Autodesk Fusion 360 part; units mm, degrees
sketch "Sketch1" plane through (0, 0, 0) normal (0, 1, 0) x (1, 0, 0)
  line L0 (4.0197, -0.419) -> (2.3727, 3.2717)
  line L1 (2.3727, 3.2717) -> (-1.647, 3.6906)
  line L2 (-1.647, 3.6906) -> (-4.0197, 0.419)
  line L3 (-4.0197, 0.419) -> (-2.3727, -3.2717)
  line L4 (-2.3727, -3.2717) -> (1.647, -3.6906)
  line L5 (1.647, -3.6906) -> (4.0197, -0.419)
  circle A0 centre (0, 0) radius 3.5
  dimension "d2" = 7
extrude "Extrude1" add sketch "Sketch1" along normal blind 2.5
sketch "Sketch2" plane through (0, 0, 0) normal (0, 1, 0) x (1, 0, 0)
  circle A0 centre (0, 0) radius 5
  dimension "d5" = 10
extrude "Extrude2" add sketch "Sketch2" against normal blind 0.5
sketch "Sketch3" plane through (0, 2.5, 0) normal (0, 1, 0) x (-1, 0, 0)
  line L0 (-1.647, 3.6906) -> (-4.0197, 0.419)
  line L1 (-4.0197, 0.419) -> (-2.3727, -3.2717)
  line L2 (-2.3727, -3.2717) -> (1.647, -3.6906)
  line L3 (1.647, -3.6906) -> (4.0197, -0.419)
  line L4 (4.0197, -0.419) -> (2.3727, 3.2717)
  line L5 (2.3727, 3.2717) -> (-1.647, 3.6906)
  circle A0 centre (0, 0) radius 3.5
  dimension "d8" = 7
extrude "Extrude3" add sketch "Sketch3" against normal blind 13 contours A0
sketch "Sketch4" plane through (0, 2.5, 0) normal (0, 1, 0) x (-1, 0, 0)
ref_plane "WorkPlane1" through (0, 1.25, 0) normal (-0.1037, 0, 0.9946) x (0.9946, 0, 0.1037)
sketch "Sketch5" plane through (0, 1.25, 0) normal (-0.1037, 0, 0.9946) x (0.9946, 0, 0.1037)
  line L0 (0, 0) -> (0, 1.25)
sketch "Sketch6" plane through (0, 1.25, 0) normal (-0.1037, 0, 0.9946) x (0.9946, 0, 0.1037)
sketch "Sketch7" plane through (0, 1.25, 0) normal (-0.1037, 0, 0.9946) x (0.9946, 0, 0.1037)
  line L0 (4.0463, 1.2672) -> (3.5, 1.2672)
  line L1 (4.0463, 1.2672) -> (4.0463, 0.9519)
  line L2 (3.5, 1.2672) -> (4.0463, 0.9519)
  line L3 (0, 6.5) -> (0, -6)
revolve "Revolve1" cut sketch "Sketch7" angle 360 about axis through (0, 7.75, 0) along (0, -1, 0)
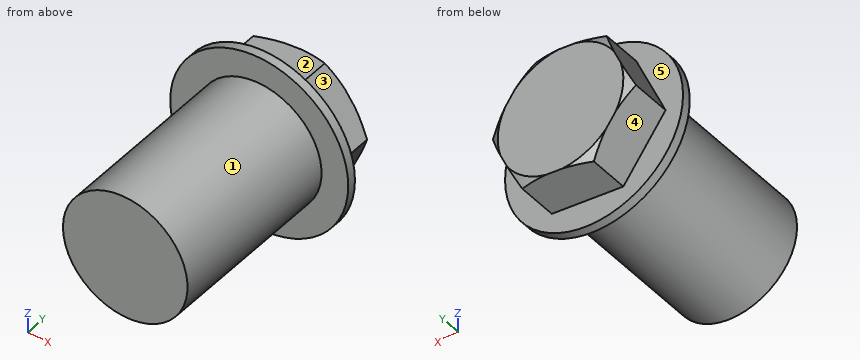
CAD build for the part. Positions are in the model's coordinates, mm. Face numbers are marked on the shaded views. A direction names the side the tool comes from. Coordinates: 2 decimals unless noted, no trailing zeros. Write each loop counter-clockwise with the first axis right and the second up, starting at its lowest first coordinate (ties: lowest second). Pieces come first, ordered by that corner, then holes. Notation, with made-up numbers: M 35.25,-31.75 L 56.25,-31.75 A11 ccw 56.25,-16.75 Z; hole C 8,-33 d8. An arc over 180 degrees is marked long. Answer as a JSON object with one key per item and string values. Group by question number.
1) Wall check: line 1 (Y direction, x = -1.75, z = 4.5); line 2 (Z direction, x = -1.25, y = -3.75); line 3 (X direction, y = -0.75, z = -2). Give the ranges that are in metal, low to high. Write a range as from..to.
2) Saw through at A-A (z = 0). Write the cut outline in (x, y), plus the area to 3 significant figures.
3) Tool access for the marked faces 1, 2, 3, 4 and 5: list every direction of +Z, -Z, +X, -X, +Y, -Y with a clear straight run to the whole face (end or side of a thin tool).
4) Pin check, flat tips, straight feed: pin 1 Ø5 at (y, z) = (-7, 0) entering from -X; pin 2 Ø3 at (x, y) = (3, -6) entering from +Z; pin 3 Ø3 at (y, z) = (-4, -1) entering from +X. Stop position of each tip, or through.
5) Saw through at B-B (y = -7.5). Write the cut outline in (x, z).
Values follow:
{
 "1": {"line 1": "y = -0.5..0", "line 2": "z = -3.27..3.27", "line 3": "x = -2.87..2.87"},
 "2": {"outline": "M -5,-0.5 L -3.5,-0.5 L -3.5,-10.5 L 3.5,-10.5 L 3.5,-0.5 L 5,-0.5 L 5,0 L 3.83,0 L 3.83,2.33 L 3.53,2.5 L -3.53,2.5 L -3.83,2.33 L -3.83,0 L -5,0 Z", "area": "94.1 mm2"},
 "3": {"face 1": "-Y", "face 2": "+Z, -X, +Y", "face 3": "+Z, +X, +Y", "face 4": "-Z, -X, +Y", "face 5": "+Y"},
 "4": {"pin 1": "stops at x = -3.5", "pin 2": "stops at z = 3.16", "pin 3": "stops at x = 3.5"},
 "5": {"outline": "C 0,0 d7"}
}
